Part model, mm, in its own coordinate system. A direction names the side the tool comes from. Round coordinates to 2 decimals unless told otherwise and drop trailing zeros. Write each loop counter-clockwise with the first axis right and the second up, starting at its lowest first coordinate (ties: lowest second). Pieces come first, ordered by that corner, then holes.
1) Saw through at C-C on z = 10.5. Write the cut outline in (x, y).
2) Which spindle directions (+Z, -Z, +X, -X, +Y, -Y) get a long thin tool onto all of the face, cutting with end or side? Do faces 5 (the flat face through (-1, -20, 1)), 6 (the cylindrical face through (24.479, -7.605, -28.034)). Say none if no direction does.
3) Saw through at B-B on x = 14. Write the cut outline in (y, z), and give its area (3 significant figures).
4) Pull direction Z, two halves, no side cores. Call faces 1 (the cylindrical face through (32.15, -4.93, -21.99)), 2 (the flat face through (-1, -10, 40)), 3 (the flat face through (5, -12, 25)), 4 (the flat face through (-1, -10, -40)): +Z half, -Z half, draft (parallel to the pull), parting line (faces both ways), or undercut.
5) Saw through at D-D on y = -6. Write the cut outline in (x, z).
6) Saw through at A-A on y = -11.75. Write the cut outline in (x, z).
7) Drill centre lines: L1, parallel to X at y = -6, z = -32; L2, parallel to Z at x = -15, y = -4.25; L3, parallel to X at y = -2.75, z = -14. Where is each one in solid material? Low to high.
8) Flat gauge pins, fed straight in: pin 1 (3 mm diameter, centred on x = 4, z = -7.5, fed in from +Y); pin 2 (10.5 mm diameter, centred on x = 25, z = -32, fed in from +Y). Where does each tip first touch, or does it go through?
```python
from build123d import *

# Parameters (mm, degrees)
F0_W     = 80
F0_H     = 80
F1_DEPTH = 20
F3_D     = 8
F3_DEPTH = 15
F3_TIP   = 2.4034424761
F5_DEPTH = 10
F7_DEPTH = 5


with BuildPart() as f1:
    # F0 (on Front) → F1 (new body)
    with BuildSketch(Plane.XZ):
        Rectangle(F0_W, F0_H)
    extrude(amount=F1_DEPTH)

    # F3
    with Locations(Plane(origin=(0, 0, 0), x_dir=(-1, 0, 0), z_dir=(0, 1, 0))):
        with Locations((-25, -32), (15, -32)):
            Hole(F3_D / 2, depth=F3_DEPTH)
            with Locations((0, 0, -(F3_DEPTH + F3_TIP / 2))):  # 118° drill point
                Cone(0, F3_D / 2, F3_TIP, mode=Mode.SUBTRACT)

    # F4 (on face) → F5 (cut)
    with BuildSketch(Plane(origin=(0, 0, 0), x_dir=(-1, 0, 0), z_dir=(0, 1, 0))):
        with BuildLine():
            ThreePointArc((25, 25), (22.0710678119, 32.0710678119), (15, 35))
            Line((15, 35), (-25, 35))
            ThreePointArc((-25, 35), (-32.0710678119, 32.0710678119), (-35, 25))
            Line((-35, 25), (-35, -15))
            ThreePointArc((-35, -15), (-32.0710678119, -22.0710678119), (-25, -25))
            Line((-25, -25), (15, -25))
            ThreePointArc((15, -25), (22.0710678119, -22.0710678119), (25, -15))
            Line((25, -15), (25, 25))
        make_face()
    extrude(amount=-F5_DEPTH, mode=Mode.SUBTRACT)

    # F6 (on face) → F7 (cut)
    with BuildSketch(Plane(origin=(0, -10, 0), x_dir=(-1, 0, 0), z_dir=(0, 1, 0))):
        with BuildLine():
            ThreePointArc((-25, -9), (-23.2426406871, -13.2426406871), (-19, -15))
            Line((-19, -15), (9, -15))
            ThreePointArc((9, -15), (13.2426406871, -13.2426406871), (15, -9))
            Line((15, -9), (15, 19))
            ThreePointArc((15, 19), (13.2426406871, 23.2426406871), (9, 25))
            Line((9, 25), (-19, 25))
            ThreePointArc((-19, 25), (-23.2426406871, 23.2426406871), (-25, 19))
            Line((-25, 19), (-25, -9))
        make_face()
    extrude(amount=-F7_DEPTH, mode=Mode.SUBTRACT)


solid = f1.part
```
Completed:
1. outline: (-40, -20) - (40, -20) - (40, 0) - (35, 0) - (35, -10) - (25, -10) - (25, -15) - (-15, -15) - (-15, -10) - (-25, -10) - (-25, 0) - (-40, 0) - close
2. face 5: +Z, -Z, +X, -X, -Y
2. face 6: +Y
3. outline: (-20, -40) - (0, -40) - (0, -25) - (-10, -25) - (-10, -15) - (-15, -15) - (-15, 25) - (-10, 25) - (-10, 35) - (0, 35) - (0, 40) - (-20, 40) - close
3. area: 800 mm2
4. face 1: undercut
4. face 2: +Z half
4. face 3: undercut
4. face 4: -Z half
5. outline: (-40, -40) - (40, -40) - (40, 40) - (-40, 40) - close; hole (-25, -15) arc R10 ccw to (-15, -25) - (25, -25) arc R10 ccw to (35, -15) - (35, 25) arc R10 ccw to (25, 35) - (-15, 35) arc R10 ccw to (-25, 25) - close; hole circle Ø8 at (-15, -32); hole circle Ø8 at (25, -32)
6. outline: (-40, -40) - (40, -40) - (40, 40) - (-40, 40) - close; hole circle Ø8 at (-15, -32); hole (-15, -9) arc R6 ccw to (-9, -15) - (19, -15) arc R6 ccw to (25, -9) - (25, 19) arc R6 ccw to (19, 25) - (-9, 25) arc R6 ccw to (-15, 19) - close; hole circle Ø8 at (25, -32)
7. L1: x = -40 to -19, -11 to 21, 29 to 40
7. L2: z = -40 to -36, -28 to -25, 35 to 40
7. L3: x = -40 to -25, 35 to 40
8. pin 1: stops at y = -15
8. pin 2: stops at y = 0
